Could you check a few things on this model? Use its own coordinates, in mm. Face numbers are marked on the shaded views. A direction names the side the tool comes from. Round coordinates to 2 decimals unless told otherwise and drop trailing zeros. Write each loop counter-clockwise with the first axis right and the second up, starting at its lowest first coordinate (ties: lowest second). Pieces come first, ordered by that corner, then holes. Notation, with made-up numbers: M 37,28 L 96,28 A14 cw 96,36 Z; hole C 82.25,12 d6. An arc over 180 degrees is marked long. One line per item, written item: value. Start each with the question number.
(1) I'm going to push flat-ended pins straight in: pin 1 Ø1.2 at (x, y) = (0.5, 8) entering from -Z; pin 2 Ø8 at (x, z) = (-15, 9.5) entering from -Y; pin 3 Ø3 at (x, z) = (6, 3) entering from -Y. Where does each tip first touch, or does it pass through?
(2) Which directions (+Z, -Z, +X, -X, +Y, -Y) give clear straight access to the entire face, cutting with the end or side of a thin tool? Please do the marked faces 1 and 2.
(3) I want a section at C-C on x = 7.5. Please give me the cut outline in (y, z).
(4) Thinking about a two-plate mould opening in X: for the marked faces 3, 4, 5 and 6, which applies, released by +X, released by -X, zero draft, split by the parting line, or undercut?
(5) If I drill on L1, parallel to X at y = -0.5, z = 3; L2, parallel to Z at x = -5, y = 8.75; L3, parallel to Y at x = -8, z = 7.25, over which ranges is the centre line in solid material (lowest first)?
(6) I want a section at B-B on z = 11.5. Please give me the cut outline in (x, y), and give its area (3 significant figures).
(7) I want a section at A-A on y = 8.25. Please give me the cut outline in (x, z).
```python
from build123d import *

# Parameters (mm, degrees)
F0_W        = 42
F0_H        = 20
F1_DEPTH    = 14
F2_T1_DEPTH = 121.3725393319
F3_T        = -1.1


# Not quite as in the source:
# - a fillet or chamfer that OpenCascade refuses, or shapes differently, is made with other operations: its cross-section is extruded or revolved along the edge and cut away or added


with BuildPart() as f1:
    # F0 (on Top) → F1 (new body)
    with BuildSketch(Plane.XY):
        Rectangle(F0_W, F0_H)
    extrude(amount=F1_DEPTH)

    # F2: fillet of radius 16 on 1 edges, made by hand

    # F2_s2 → F2_t1 (cut)
    with BuildSketch(Plane.YZ.offset(-60.686269666)):
        with BuildLine():
            ThreePointArc((-10, 0), (-4.7084973779, 10), (5.8745078664, 14))
            Line((5.8745078664, 14), (-10, 14))
            Line((-10, 14), (-10, 0))
        make_face()
    extrude(amount=F2_T1_DEPTH, mode=Mode.SUBTRACT)

    # F3
    f3_openings = [f1.faces().sort_by_distance(p)[0] for p in [
        (0, 10, 7),
        (0, 0, 0),
    ]]
    offset(amount=F3_T, openings=f3_openings)


solid = f1.part
```
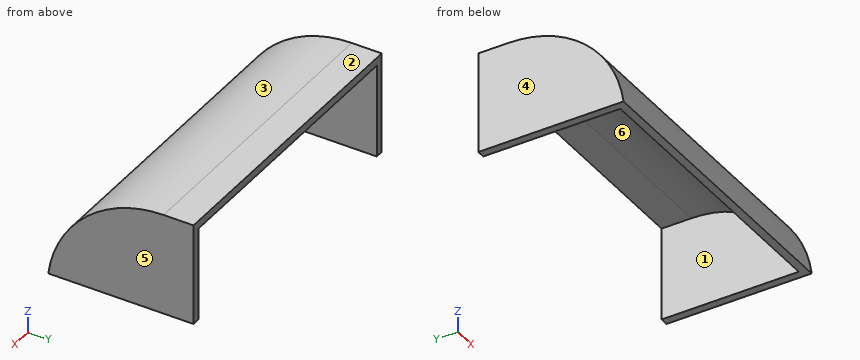
Found:
1. pin 1: stops at z = 12.9
1. pin 2: stops at y = -8.26
1. pin 3: stops at y = -9.74
2. face 1: -Z, +Y
2. face 2: +Z, +X, -X, +Y, -Y
3. outline: M -10,0 L -8.89,0 A14.9 cw 5.87,12.9 L 10,12.9 L 10,14 L 5.87,14 A16 ccw Z
4. face 3: zero draft
4. face 4: released by -X
4. face 5: released by +X
4. face 6: undercut
5. L1: x = -21 to -19.9, 19.9 to 21
5. L2: z = 12.9 to 14
5. L3: y = -7.18 to -5.81
6. outline: M -21,-2.71 L 21,-2.71 L 21,10 L 19.9,10 L 19.9,-0.43 L -19.9,-0.43 L -19.9,10 L -21,10 Z
6. area: 119 mm²
7. outline: M -21,0 L -19.9,0 L -19.9,12.9 L 19.9,12.9 L 19.9,0 L 21,0 L 21,14 L -21,14 Z
